For this review, take the finished solid that the model builds, in its own axes (mm). A direction names the side the tool comes from. Give positions to 0.01 mm unless a question says otherwise; leave off trailing zeros. Loops run counter-clockwise (first coordinate to the right, second up) from the corner with the lowest first, then second, coordinate; pieces in that order, holes last. Notation, with made-up numbers: (-39, 34.25) - (-14, 34.25) arc R23 ccw to (-14, 55.25) - close; hole circle Ø7 at (43.5, 4). An arc over 180 degrees is marked (long way). Answer in a Markdown table with one row per item.
Autodesk Inventor part; units mm, degrees
ref_plane "YZ Plane" through (0, 0, 0) normal (1, 0, 0) x (0, 1, 0)
ref_plane "XZ Plane" through (0, 0, 0) normal (0, 1, 0) x (-1, 0, 0)
ref_plane "XY Plane" through (0, 0, 0) normal (0, 0, 1) x (1, 0, 0)
sketch "Sketch1" plane through (0, 0, 0) normal (0, 1, 0) x (-1, 0, 0)
  line L0 (-68.199, -71.3867) -> (68.199, -71.3867)
  line L1 (68.199, -71.3867) -> (68.199, 71.3867)
  line L2 (68.199, 71.3867) -> (-68.199, 71.3867)
  line L3 (-68.199, 71.3867) -> (-68.199, -71.3867)
  line L4 (-68.199, -71.3867) -> (68.199, 71.3867) construction
  line L5 (68.199, -71.3867) -> (-68.199, 71.3867) construction
  point P0 (0, 0)
  dimension "d0" = 136.398
  dimension "d1" = 142.7734
extrude "Extrusion1" add sketch "Sketch1" along normal blind 6.35
sketch "Sketch2" plane through (0, 6.35, 0) normal (0, 1, 0) x (1, 0, 0)
  line L0 (-68.199, 71.3867) -> (-68.199, -71.3867)
  line L1 (-68.199, -71.3867) -> (68.199, -71.3867)
  line L2 (68.199, -71.3867) -> (68.199, 71.3867)
  line L3 (-59.436, -54.7751) -> (-59.436, 54.7497) construction
  line L4 (-59.436, 54.7497) -> (23.114, 54.7497) construction
  line L5 (23.114, 54.7497) -> (23.114, -54.7751) construction
  line L6 (23.114, -54.7751) -> (-59.436, -54.7751) construction
  line L7 (68.199, 71.3867) -> (-68.199, 71.3867)
  point P0 (0, 0)
  dimension "d4" = 8.763
  dimension "d5" = 16.6116
  dimension "d8" = 82.55
  dimension "d9" = 109.5248
  dimension "d17" = 16.637
hole "Hole1" at (-59.436, 6.35, -54.7497) at (23.114, 6.35, -54.7497) at (23.114, 6.35, 54.7751) at (-59.436, 6.35, 54.7751) direction (0, -1, 0) diameter 6.7818 end through all
sketch "Sketch3" plane through (0, 6.35, 0) normal (0, 1, 0) x (1, 0, 0)
  line L0 (59.563, -45.9867) -> (19.1008, -45.9867)
  line L1 (59.563, -25.6667) -> (59.563, -45.9867)
  line L2 (19.1008, -25.6667) -> (59.563, -25.6667)
  line L3 (19.1008, -45.9867) -> (19.1008, -25.6667)
  point P0 (0, 0)
extrude "Extrusion2" cut sketch "Sketch3" against normal up to next
properties part number "loader_frame"
1. We need section D-D, the plane z = 56.5. Give the boundary of the cut face in (x, y).
Values:
| item | result |
|---|---|
| outline | (-68.2, 0) - (-62.36, 0) - (-62.36, 6.35) - (-68.2, 6.35) - close; (-56.52, 0) - (20.19, 0) - (20.19, 6.35) - (-56.52, 6.35) - close; (26.03, 0) - (68.2, 0) - (68.2, 6.35) - (26.03, 6.35) - close |
2. We need section C-C, the plane y = 3.5. Give the boundary of the cut face in (x, z), and give its area (3 significant figures).
Values:
| item | result |
|---|---|
| outline | (-68.2, -71.39) - (68.2, -71.39) - (68.2, 71.39) - (-68.2, 71.39) - close; hole circle Ø6.78 at (-59.44, -54.75); hole circle Ø6.78 at (-59.44, 54.78); hole (19.1, 25.67) - (59.56, 25.67) - (59.56, 45.99) - (19.1, 45.99) - close; hole circle Ø6.78 at (23.11, -54.75); hole circle Ø6.78 at (23.11, 54.78) |
| area | 18,500 mm^2 |
3. We need section A-A, the plane x = 32.5. Give the boundary of the cut face in (y, z).
Values:
| item | result |
|---|---|
| outline | (0, -71.39) - (6.35, -71.39) - (6.35, 25.67) - (0, 25.67) - close; (0, 45.99) - (6.35, 45.99) - (6.35, 71.39) - (0, 71.39) - close |
4. Mouldability with a two-part tool opening along X and no side actions: class faces 3 (the face through (1, 0, 1)), 4 (the face through (26.424, 3.131, -55.485)), 5 (the face through (68.199, 3, 1)) as released by +X, released by -X, zero draft, split by the parting line, or undercut.
Values:
| item | result |
|---|---|
| face 3 | zero draft |
| face 4 | undercut |
| face 5 | released by +X |
5. For faces 1 (the face through (19.101, 3, 36)), 2 (the face through (1, 6.35, 1)), list the 3-axis set-ups (+Z, -Z, +X, -X, +Y, -Y) from which the entire face can be reached by the end or side of a thin tool; tool diameter is ignored.
Values:
| item | result |
|---|---|
| face 1 | +Y, -Y |
| face 2 | +Z, -Z, +X, -X, +Y |
6. We need section B-B, the plane z = -54.5. Give the boundary of the cut face in (x, y), and give its area (3 significant figures).
Values:
| item | result |
|---|---|
| outline | (-68.2, 0) - (-62.82, 0) - (-62.82, 6.35) - (-68.2, 6.35) - close; (-56.05, 0) - (19.73, 0) - (19.73, 6.35) - (-56.05, 6.35) - close; (26.5, 0) - (68.2, 0) - (68.2, 6.35) - (26.5, 6.35) - close |
| area | 780 mm^2 |
7. Clearance check with a flat-ended pin moving along its axis: pin 1 (8 mm diameter, centred on x = 23.11, z = 54.78, fed in from +Y). State where the tip first meets the part, or that it passes through.
Values:
| item | result |
|---|---|
| pin 1 | stops at y = 6.35 |
8. Wall thickness on line 1 (Z direction, x = -59, y = 3.5); line 2 (Z direction, x = 31, y = 0.5); line 3 (X direction, y = 2.75, z = 33.5): over which ranges is each line inside the solid? List them lowest first. Write a range as [from, to].
Values:
| item | result |
|---|---|
| line 1 | z = [-71.39, -58.11], [-51.39, 51.41], [58.14, 71.39] |
| line 2 | z = [-71.39, 25.67], [45.99, 71.39] |
| line 3 | x = [-68.2, 19.1], [59.56, 68.2] |
